from build123d import *

# Parameters (mm, degrees)
SKETCH1_W             = 42
SKETCH1_H             = 30
BOSS_EXTRUDE1_DEPTH   = 8
BOSS_EXTRUDE1_2_DEPTH = 8
BOSS_EXTRUDE2_DEPTH   = 30
SKETCH2_R             = 2.5
CUT_EXTRUDE1_DEPTH    = 8
SKETCH3_R             = 2.75
CUT_EXTRUDE2_DEPTH    = 10


with BuildPart() as part:
    # Sketch1 → Boss-Extrude1 (new body)
    with BuildSketch(Plane.XY):
        with Locations((21, 133)):
            Rectangle(SKETCH1_W, SKETCH1_H)
    extrude(amount=BOSS_EXTRUDE1_DEPTH)



with BuildPart() as body_2:
    # Sketch1 → Boss-Extrude1 2 (new body)
    with BuildSketch(Plane.XY):
        with Locations((21, 15)):
            Rectangle(SKETCH1_W, SKETCH1_H)
    extrude(amount=BOSS_EXTRUDE1_2_DEPTH)


with BuildPart() as part_1:
    add(part.part)

    add(body_2.part)  # Boss-Extrude2 merges body 2
    # Sketch1_3 → Boss-Extrude2 (add)
    with BuildSketch(Plane.XY):
        Polygon((42, 30), (42, 0), (52, 0), (52, 148), (42, 148), (42, 118), align=None)
    extrude(amount=BOSS_EXTRUDE2_DEPTH)

    # Sketch2 → Cut-Extrude1 (cut)
    with BuildSketch(Plane.XY.offset(8)):
        with Locations((8, 133)):
            Circle(SKETCH2_R)
        with Locations((34, 133)):
            Circle(SKETCH2_R)
        with Locations((34, 15)):
            Circle(SKETCH2_R)
        with Locations((8, 15)):
            Circle(SKETCH2_R)
    extrude(amount=-CUT_EXTRUDE1_DEPTH, mode=Mode.SUBTRACT)

    # Sketch3 → Cut-Extrude2 (cut)
    with BuildSketch(Plane(origin=(52, 0, 0), x_dir=(0, 0, -1), z_dir=(1, 0, 0))):
        with Locations((-20, 138.3)):
            Circle(SKETCH3_R)
        with Locations((-20, 106.3)):
            Circle(SKETCH3_R)
        with Locations((-20, 41.2)):
            Circle(SKETCH3_R)
        with Locations((-20, 9.2)):
            Circle(SKETCH3_R)
    extrude(amount=-CUT_EXTRUDE2_DEPTH, mode=Mode.SUBTRACT)


solid = part_1.part
The model under review builds one solid part; all positions refer to its coordinate system, in mm. A direction names the side the tool comes from. Round coordinates to 2 decimals unless told otherwise and drop trailing zeros. Loops run counter-clockwise (first coordinate to the right, second up) from the corner with the lowest first, then second, coordinate; pieces in that order, holes last. Notation, with made-up numbers: (22.25, 57) -> (71.25, 57) arc R12 ccw to (71.25, 69) -> close; hole circle Ø2 at (-1.75, 38). An arc over 180 degrees is marked (long way). Return JSON: item names as keys, results as strings.
(1) The part is to be moulded in two halves that separate along Z. For faces 3 (the flat face through (21, 133, 8)), 4 (the flat face through (21, 30, 4)), 5 (the cylindrical face through (47.07, 38.515, 20.596)), say which applies: released by +Z, released by -Z, zero draft, split by the parting line, or undercut.
Solved:
{"face 3": "released by +Z", "face 4": "zero draft", "face 5": "undercut"}
(2) Add section A-A on z = 20. Write out the cut boundary in (x, y).
Solved:
{"outline": "(42, 0) -> (52, 0) -> (52, 6.45) -> (42, 6.45) -> close; (42, 11.95) -> (52, 11.95) -> (52, 38.45) -> (42, 38.45) -> close; (42, 43.95) -> (52, 43.95) -> (52, 103.55) -> (42, 103.55) -> close; (42, 109.05) -> (52, 109.05) -> (52, 135.55) -> (42, 135.55) -> close; (42, 141.05) -> (52, 141.05) -> (52, 148) -> (42, 148) -> close"}
(3) For line 1 (Y direction, x = 8, z = 6); line 2 (Y direction, x = 44.5, z = 20); line 3 (Y direction, x = 28.5, z = 5), list the stretches that pass through material, from the lowest coordinate up.
Solved:
{"line 1": "0 to 12.5, 17.5 to 30, 118 to 130.5, 135.5 to 148", "line 2": "0 to 6.45, 11.95 to 38.45, 43.95 to 103.55, 109.05 to 135.55, 141.05 to 148", "line 3": "0 to 30, 118 to 148"}
(4) Add section B-B on y = 138.3. Write out the cut boundary in (x, z), plus the area to 3 significant figures.
Solved:
{"outline": "(0, 0) -> (52, 0) -> (52, 17.25) -> (42, 17.25) -> (42, 8) -> (0, 8) -> close; (42, 22.75) -> (52, 22.75) -> (52, 30) -> (42, 30) -> close", "area": "581 mm2"}
(5) Add section C-C on z = 3. Write out the cut boundary in (x, y).
Solved:
{"outline": "(0, 0) -> (52, 0) -> (52, 148) -> (0, 148) -> (0, 118) -> (42, 118) -> (42, 30) -> (0, 30) -> close; hole circle Ø5 at (8, 15); hole circle Ø5 at (8, 133); hole circle Ø5 at (34, 15); hole circle Ø5 at (34, 133)"}
(6) For pin 1 (9 mm diameter, centred on y = 49, z = 13, fed in from -X); pin 2 (15 mm diameter, centred on x = 26, y = 130.5, fed in from +Z), all flat-tipped, find the tip position at first contact; note any pin that passes through.
Solved:
{"pin 1": "x = 42", "pin 2": "z = 8"}
(7) For faces 1 (the flat face through (42, 75, 15)), 2 (the flat face through (37, 0, 5)), list the 3-axis set-ups (+Z, -Z, +X, -X, +Y, -Y) from which the entire face can be reached by the end or side of a thin tool; tool diameter is ignored.
Solved:
{"face 1": "+Z, -X", "face 2": "+Z, -Z, +X, -X, -Y"}
(8) Add section D-D on x = 8. Write out the cut boundary in (y, z), plus the area to 3 significant figures.
Solved:
{"outline": "(0, 0) -> (12.5, 0) -> (12.5, 8) -> (0, 8) -> close; (17.5, 0) -> (30, 0) -> (30, 8) -> (17.5, 8) -> close; (118, 0) -> (130.5, 0) -> (130.5, 8) -> (118, 8) -> close; (135.5, 0) -> (148, 0) -> (148, 8) -> (135.5, 8) -> close", "area": "400 mm2"}
